Answer from the drawing. Dimensions are ordinates in mm from the lowest x, y and z of the part. A direction names the side the tool comes from. Coordinates: 2 decimals unless noted, no trailing zeros. Loops run counter-clockwise (first coordinate to the right, second up) from the corner with the lowest first, then second, coordinate; pieces in that order, holes last. Notation, with made-up numbers: (-6.75, 32) -> (36.25, 32) arc R30 ccw to (36.25, 61) -> close; hole circle Ø2 at (43, -7). An arc over 180 degrees is marked (long way). Use a Markdown table: item, result.
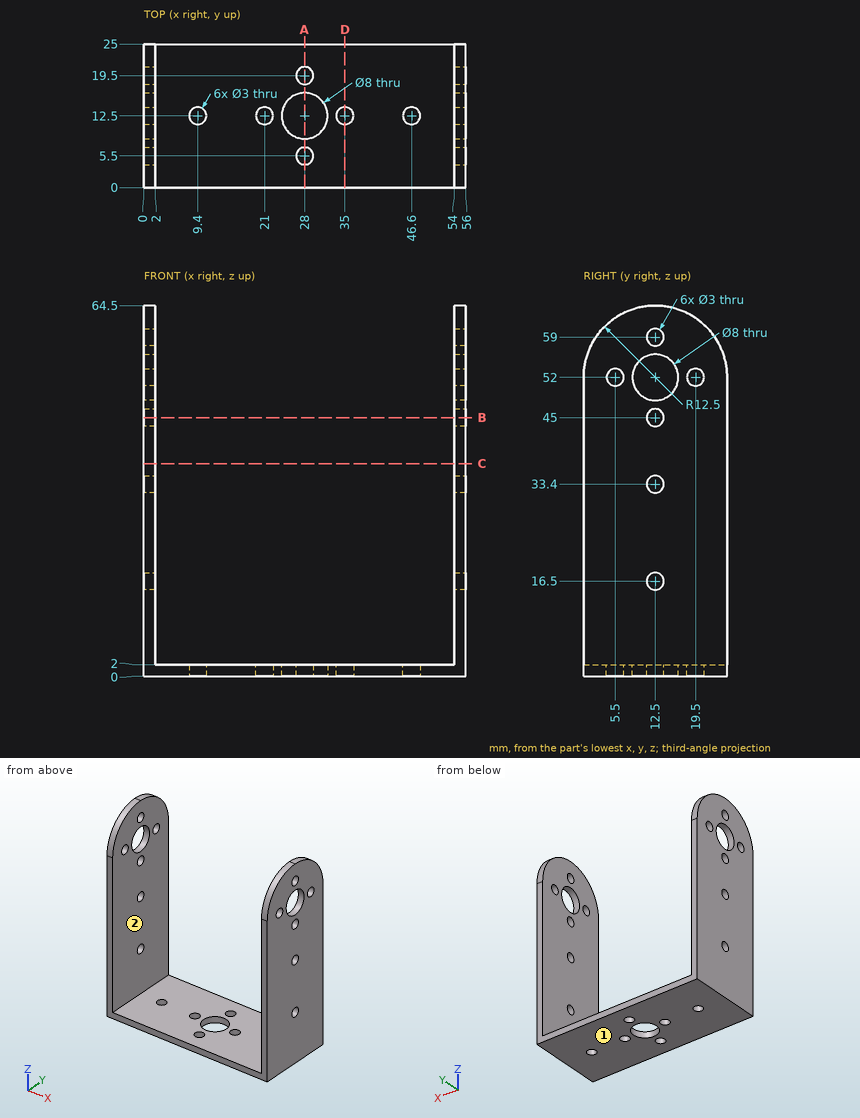
Q1. Given pin 1 Ø12.5 at (x, y) = (29.5, 11.5) entering from +Z; pin 2 Ø2.5 at (y, z) = (19.5, 52) entering from +X, each flat-ended and moving along its own axis, determine where each tip first touches the part or whether it passes through.
Solved:
| item | result |
|---|---|
| pin 1 | z = 2 |
| pin 2 | through |
Q2. For the marked faces 1 and 2, determine the directions among +Z, -Z, +X, -X, +Y, -Y from which every point of the face is accessible in a straight line to the end or side of a thin tool.
Solved:
| item | result |
|---|---|
| face 1 | -Z, +X, -X, +Y, -Y |
| face 2 | +Z, +Y, -Y |
Q3. Section B-B on z = 45 is taken. Determine the outline of the cut face in (x, y), and give its area (3 significant figures).
Solved:
| item | result |
|---|---|
| outline | (0, 0) -> (2, 0) -> (2, 11) -> (0, 11) -> close; (0, 14) -> (2, 14) -> (2, 25) -> (0, 25) -> close; (54, 0) -> (56, 0) -> (56, 11) -> (54, 11) -> close; (54, 14) -> (56, 14) -> (56, 25) -> (54, 25) -> close |
| area | 88.0 mm² |
Q4. Section C-C on z = 37 is taken. Determine the outline of the cut face in (x, y).
Solved:
| item | result |
|---|---|
| outline | (0, 0) -> (2, 0) -> (2, 25) -> (0, 25) -> close; (54, 0) -> (56, 0) -> (56, 25) -> (54, 25) -> close |
Q5. Section D-D on x = 35 is taken. Determine the outline of the cut face in (y, z), and give its area (3 significant figures).
Solved:
| item | result |
|---|---|
| outline | (0, 0) -> (11, 0) -> (11, 2) -> (0, 2) -> close; (14, 0) -> (25, 0) -> (25, 2) -> (14, 2) -> close |
| area | 44.0 mm² |
Q6. Section A-A on x = 28 is taken. Determine the outline of the cut face in (y, z).
Solved:
| item | result |
|---|---|
| outline | (0, 0) -> (4, 0) -> (4, 2) -> (0, 2) -> close; (7, 0) -> (8.5, 0) -> (8.5, 2) -> (7, 2) -> close; (16.5, 0) -> (18, 0) -> (18, 2) -> (16.5, 2) -> close; (21, 0) -> (25, 0) -> (25, 2) -> (21, 2) -> close |
Q7. Consider line 1 (X direction, y = 19.25, z = 54.5); line 2 (Y direction, x = 21, z = 1.55); line 3 (Z direction, x = 3, y = 13.5). Determine where each line is inside the solid, lowest interval first. Write a range as [from, to].
Solved:
| item | result |
|---|---|
| line 1 | [0, 2], [54, 56] |
| line 2 | [0, 11], [14, 25] |
| line 3 | [0, 2] |
